from build123d import *

# Parameters (mm, degrees)
SKETCH1_W           = 31.75
SKETCH1_H           = 50.8
BOSS_EXTRUDE1_DEPTH = 13.081
CUT_EXTRUDE1_REACH  = 15.081
SKETCH2_R           = 3.175


with BuildPart() as part:
    # Sketch1 → Boss-Extrude1 (new body)
    with BuildSketch(Plane.XY):
        with Locations((15.875, 25.4)):
            Rectangle(SKETCH1_W, SKETCH1_H)
    extrude(amount=BOSS_EXTRUDE1_DEPTH)

    # Sketch2 → Cut-Extrude1 (cut, up to next)
    with BuildSketch(Plane.XY.offset(13.081), mode=Mode.PRIVATE) as cut_extrude1_sk1:
        with Locations((25.4, 34.925)):
            Circle(SKETCH2_R)
    cut_extrude1_tool1 = extrude(cut_extrude1_sk1.sketch, amount=-CUT_EXTRUDE1_REACH, mode=Mode.PRIVATE) & part.part
    add(cut_extrude1_tool1.solids().sort_by_distance((25.4, 34.925, 13.081))[0], mode=Mode.SUBTRACT)
    # Sketch2 → Cut-Extrude1 (cut, up to next)
    with BuildSketch(Plane.XY.offset(13.081), mode=Mode.PRIVATE) as cut_extrude1_sk2:
        with Locations((6.35, 34.925)):
            Circle(SKETCH2_R)
    cut_extrude1_tool2 = extrude(cut_extrude1_sk2.sketch, amount=-CUT_EXTRUDE1_REACH, mode=Mode.PRIVATE) & part.part
    add(cut_extrude1_tool2.solids().sort_by_distance((6.35, 34.925, 13.081))[0], mode=Mode.SUBTRACT)
    # Sketch2 → Cut-Extrude1 (cut, up to next)
    with BuildSketch(Plane.XY.offset(13.081), mode=Mode.PRIVATE) as cut_extrude1_sk3:
        with Locations((6.35, 15.875)):
            Circle(SKETCH2_R)
    cut_extrude1_tool3 = extrude(cut_extrude1_sk3.sketch, amount=-CUT_EXTRUDE1_REACH, mode=Mode.PRIVATE) & part.part
    add(cut_extrude1_tool3.solids().sort_by_distance((6.35, 15.875, 13.081))[0], mode=Mode.SUBTRACT)
    # Sketch2 → Cut-Extrude1 (cut, up to next)
    with BuildSketch(Plane.XY.offset(13.081), mode=Mode.PRIVATE) as cut_extrude1_sk4:
        with Locations((25.4, 15.875)):
            Circle(SKETCH2_R)
    cut_extrude1_tool4 = extrude(cut_extrude1_sk4.sketch, amount=-CUT_EXTRUDE1_REACH, mode=Mode.PRIVATE) & part.part
    add(cut_extrude1_tool4.solids().sort_by_distance((25.4, 15.875, 13.081))[0], mode=Mode.SUBTRACT)


solid = part.part
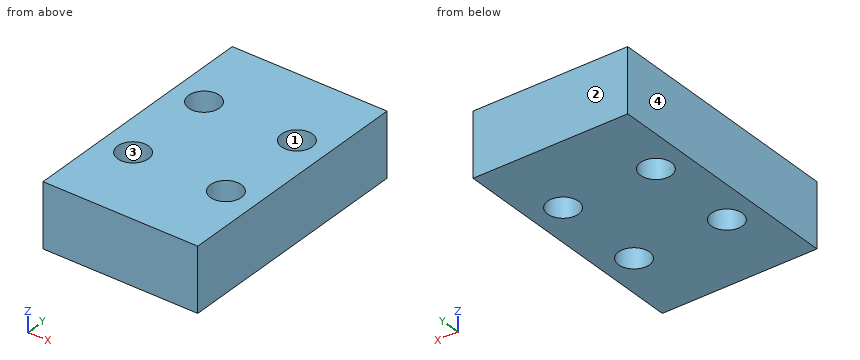
Can you work these out from the model? Positions are in its coordinate system, mm. Face numbers are marked on the shaded views. Coordinates: 2 decimals unless noted, no trailing zeros. Order: outer loops, then holes, each group sorted by start corner. A loop starts at its lowest first (then second) coordinate and runs counter-clockwise, first axis right, second up. Notation, with made-up numbers: (14, 70.25) - (55, 70.25) arc R31 cw to (55, 109.25) - close; hole circle Ø6 at (-35.5, 41.25). An arc over 180 degrees is marked (long way). Answer as a JSON object with one key per item and string values. Group by question number.
Q1. Imagine slicing it at A-A (x = 25.4). Please give me the cut outline in (y, z).
Q2. I need wall thicknesses on line 1 (Y direction, x = 25.4, z = 5.75); line 2 (X direction, y = 17.5, z = 2.5); line 3 (Y direction, x = 8, z = 8.5). Which ranges of each line are inside material? Lowest first, please. Write a range as from..to.
Q3. We'd pull the mould along Y, two halves only. Please class the marked faces 1, 2, 3 and 4: +Y half, -Y half, draft (parallel to the pull), parting line (faces both ways), or undercut.
Q4. Imagine slicing it at C-C (y = 32.5). Please give me the cut outline in (x, z).
Q5. Imagine slicing it at B-B (z = 1.25). Please give me the cut outline in (x, y) (3 decimals).
Determined:
{
 "1": {"outline": "(0, 0) - (12.7, 0) - (12.7, 13.08) - (0, 13.08) - close; (19.05, 0) - (31.75, 0) - (31.75, 13.08) - (19.05, 13.08) - close; (38.1, 0) - (50.8, 0) - (50.8, 13.08) - (38.1, 13.08) - close"},
 "2": {"line 1": "y = 0..12.7, 19.05..31.75, 38.1..50.8", "line 2": "x = 0..3.62, 9.08..22.67, 28.13..31.75", "line 3": "y = 0..13.16, 18.59..32.21, 37.64..50.8"},
 "3": {"face 1": "undercut", "face 2": "+Y half", "face 3": "undercut", "face 4": "draft"},
 "4": {"outline": "(0, 0) - (4.3, 0) - (4.3, 13.08) - (0, 13.08) - close; (8.4, 0) - (23.35, 0) - (23.35, 13.08) - (8.4, 13.08) - close; (27.45, 0) - (31.75, 0) - (31.75, 13.08) - (27.45, 13.08) - close"},
 "5": {"outline": "(0, 0) - (31.75, 0) - (31.75, 50.8) - (0, 50.8) - close; hole circle Ø6.35 at (6.35, 15.875); hole circle Ø6.35 at (6.35, 34.925); hole circle Ø6.35 at (25.4, 15.875); hole circle Ø6.35 at (25.4, 34.925)"}
}
